Design review of the part built by this model. Coordinates are the model's own, in mm. A direction names the side the tool comes from. Give positions to 0.01 mm unless a question says otherwise; leave off trailing zeros. Order: outer loops, then holes, each group sorted by start corner. A loop starts at its lowest first (then second) coordinate and runs counter-clockwise, first axis right, second up. Notation, with made-up numbers: (33.25, 81.5) -> (40.25, 81.5) arc R15 ccw to (40.25, 105.5) -> close; hole circle Ø8 at (73.5, -18). An arc over 180 degrees is marked (long way). Return JSON: item names as keys, results as strings.
```python
from build123d import *

# Parameters (mm, degrees)
ESTRUSIONE_ESTRUSIONE1_DEPTH      = 30
ESTRUSIONE_ESTRUSIONE1_DEPTH_BACK = 55
SCHIZZO1_R                        = 25
SCHIZZO1_R_2                      = 20
ESTRUSIONE_ESTRUSIONE2_DEPTH      = 10
ESTRUSIONE_ESTRUSIONE3_DEPTH      = 10
ESTRUSIONE_ESTRUSIONE5_DEPTH      = 42.5
TAGLIO_ESTRUSIONE1_DEPTH          = 26.5
SCHIZZO3D5_R                      = 2.5
TAGLIO_ESTRUSIONE2_DEPTH          = 35.5
SCHIZZO3D6_R                      = 4
TAGLIO_ESTRUSIONE3_DEPTH          = 3
ESTRUSIONE_ESTRUSIONE10_DEPTH     = 5
TAGLIO_ESTRUSIONE4_START          = -14
TAGLIO_ESTRUSIONE4_DEPTH          = 14
TAGLIO_ESTRUSIONE7_DEPTH          = 3
ESTRUSIONE_ESTRUSIONE11_START     = 30
ESTRUSIONE_ESTRUSIONE11_OUTLINE_R = 4
ESTRUSIONE_ESTRUSIONE11_DEPTH     = 10
ESTRUSIONE_ESTRUSIONE12_DEPTH     = 10
ESTRUSIONE_ESTRUSIONE13_DEPTH     = 10
ESTRUSIONE_ESTRUSIONE14_DEPTH     = 10
TAGLIO_ESTRUSIONE11_DEPTH         = 80
SCHIZZO3D17_R                     = 4
TAGLIO_ESTRUSIONE12_DEPTH         = 3
TAGLIO_ESTRUSIONE13_START         = 30
TAGLIO_ESTRUSIONE13_OUTLINE_R     = 2.5
TAGLIO_ESTRUSIONE13_DEPTH         = 7
TAGLIO_ESTRUSIONE14_START         = -55
TAGLIO_ESTRUSIONE14_OUTLINE_R     = 25
TAGLIO_ESTRUSIONE14_OUTLINE_R_2   = 20
TAGLIO_ESTRUSIONE14_DEPTH         = 20


# Read off the part's stored shape, not the designer's step: Estrusione-Estrusione11, Taglio-Estrusione13, Taglio-Estrusione14
with BuildPart() as part:
    # Schizzo1 → Estrusione-Estrusione1 (new, two sides: drawn at the far end of the back side and taken through both)
    with BuildSketch(Plane.XY.offset(-ESTRUSIONE_ESTRUSIONE1_DEPTH_BACK)):
        Circle(SCHIZZO1_R)
        Circle(SCHIZZO1_R_2, mode=Mode.SUBTRACT)
    extrude(amount=ESTRUSIONE_ESTRUSIONE1_DEPTH + ESTRUSIONE_ESTRUSIONE1_DEPTH_BACK)

    # Schizzo3D1 → Estrusione-Estrusione2 (add)
    with BuildSketch(Plane(origin=(-37.75, 73.5, 30), x_dir=(0.4568693936855125, -0.889533786381064, 0), z_dir=(0, 0, -1))):
        Polygon((0, 0), (34.493639223, -67.159800872), (75.600538561, -73.870637396), (146.763241471, -37.321085901), (165.255105821, 0), (130.761466598, 67.159800872), (89.654567261, 73.870637396), (18.49186435, 37.321085901), align=None)
    extrude(amount=-ESTRUSIONE_ESTRUSIONE2_DEPTH)

    # Schizzo3D2 → Estrusione-Estrusione3 (add)
    with BuildSketch(Plane(origin=(62.5, 0, 30), x_dir=(-0.9968152785361251, -0.07974522228289001, 0), z_dir=(0, 0, 1))):
        Polygon((0, 0), (0.797452223, 9.968152785), (5.781528616, 9.569426674), (4.984076393, -0.398726111), align=None)
        Polygon((125.39936204, 0), (120.415285647, 0.398726111), (119.617833424, -9.569426674), (124.601909817, -9.968152785), align=None)
    extrude(amount=-ESTRUSIONE_ESTRUSIONE3_DEPTH)

    # Schizzo3D3 → Estrusione-Estrusione5 (add)
    with BuildSketch(Plane(origin=(35.227450684, -68.5, 30), x_dir=(-0.9974912873801348, -0.0707893466612134, 0), z_dir=(0, 0, 1))):
        Polygon((0, 0), (70.278150268, -4.987456437), (70.632097001, 0), (0.353946733, 4.987456437), align=None)
    extrude(amount=-ESTRUSIONE_ESTRUSIONE5_DEPTH)

    # Schizzo3D4 → Taglio-Estrusione1 (cut)
    with BuildSketch(Plane(origin=(32.75, -68.5, -12.5), x_dir=(-1, 0, 0), z_dir=(0, 1, 0))):
        with BuildLine():
            Line((0, 0), (65.5, 0))
            ThreePointArc((65.5, 0), (32.75, 32.75), (0, 0))
        make_face()
    extrude(amount=-TAGLIO_ESTRUSIONE1_DEPTH, mode=Mode.SUBTRACT)

    # Schizzo3D5 → Taglio-Estrusione2 (cut)
    with BuildSketch(Plane(origin=(-52.5, 33.353317087, 40), x_dir=(0.8440673996564301, -0.5362370975951146, 0), z_dir=(0, 0, -1))):
        with Locations(Location((0, 0, 0), (0, 0, 147.572152721))):
            Circle(SCHIZZO3D5_R)
        with Locations(Location((88.627076964, -56.304895247, 0), (0, 0, 147.572152721))):
            Circle(SCHIZZO3D5_R)
        with Locations(Location((124.397648864, 0, 0), (0, 0, 147.572152721))):
            Circle(SCHIZZO3D5_R)
        with Locations(Location((35.7705719, 56.304895247, 0), (0, 0, 147.572152721))):
            Circle(SCHIZZO3D5_R)
    extrude(amount=TAGLIO_ESTRUSIONE2_DEPTH, mode=Mode.SUBTRACT)

    # Schizzo3D6 → Taglio-Estrusione3 (cut)
    with BuildSketch(Plane(origin=(0, 73.5, 40), x_dir=(0, -1, 0), z_dir=(0, 0, -1))):
        with Locations(Location((40.146682913, 52.5, 0), (0, 0, 270))):
            Circle(SCHIZZO3D6_R)
        with Locations(Location((40.146682913, -52.5, 0), (0, 0, 270))):
            Circle(SCHIZZO3D6_R)
        with Locations(Location((106.853317087, -52.5, 0), (0, 0, 270))):
            Circle(SCHIZZO3D6_R)
        with Locations(Location((106.853317087, 52.5, 0), (0, 0, 270))):
            Circle(SCHIZZO3D6_R)
    extrude(amount=TAGLIO_ESTRUSIONE3_DEPTH, mode=Mode.SUBTRACT)

    # Schizzo3D7 → Estrusione-Estrusione10 (add)
    with BuildSketch(Plane(origin=(35.227450684, -73.5, -12.5), x_dir=(-0.8117651174974726, 0, 0.5839840700004706), z_dir=(0, 1, 0))):
        with BuildLine():
            Line((0, 0), (2.011108045, -1.446791734))
            ThreePointArc((2.011108045, -1.446791734), (47.721893936, 6.013037572), (55.181723242, -39.697748319))
            Line((55.181723242, -39.697748319), (57.192831287, -41.144540052))
            Line((57.192831287, -41.144540052), (82.012154262, -6.644522559))
            Line((82.012154262, -6.644522559), (84.059871804, -8.117651175))
            Line((84.059871804, -8.117651175), (89.899712504, 0))
            Line((89.899712504, 0), (28.611446133, 44.090797285))
            Line((28.611446133, 44.090797285), (22.771605433, 35.97314611))
            Line((22.771605433, 35.97314611), (24.819322975, 34.500017494))
            Line((24.819322975, 34.500017494), (0, 0))
        make_face()
    extrude(amount=-ESTRUSIONE_ESTRUSIONE10_DEPTH)

    # Schizzo3D8 → Taglio-Estrusione4 (cut)
    with BuildSketch(Plane(origin=(0, -78.5, 20.25), x_dir=(-0.707106781186551, 0, -0.7071067811865441), z_dir=(0, -1, 0)).offset(TAGLIO_ESTRUSIONE4_START)):
        with BuildLine():
            ThreePointArc((0, 46.315494168), (-0.707106781, -0.707106781), (46.315494168, 0))
            ThreePointArc((46.315494168, 0), (0, 0), (0, 46.315494168))
        make_face()
    extrude(amount=TAGLIO_ESTRUSIONE4_DEPTH, mode=Mode.SUBTRACT)

    # Schizzo3D9 → Taglio-Estrusione7 (cut)
    with BuildSketch(Plane(origin=(35.227450684, -68.5, -12.5), x_dir=(-0.8562730712113632, 0, 0.5165234046180869), z_dir=(0, -1, 0))):
        with BuildLine():
            Line((0, 0), (2.121374306, 1.279661262))
            ThreePointArc((2.121374306, 1.279661262), (13.749394894, 45.407843828), (58.20726047, 35.111944264))
            Line((58.20726047, 35.111944264), (60.328634776, 36.391605526))
            Line((60.328634776, 36.391605526), (82.280879472, 0))
            Line((82.280879472, 0), (21.952244696, -36.391605526))
            Line((21.952244696, -36.391605526), (0, 0))
        make_face()
    extrude(amount=TAGLIO_ESTRUSIONE7_DEPTH, mode=Mode.SUBTRACT)

    # Estrusione-Estrusione11 outline → Estrusione-Estrusione11 (add)
    with BuildSketch(Plane.XY.offset(ESTRUSIONE_ESTRUSIONE11_START)):
        with Locations((52.5, -33.353317087)):
            Circle(ESTRUSIONE_ESTRUSIONE11_OUTLINE_R)
        with Locations((-52.5, -33.353317087)):
            Circle(ESTRUSIONE_ESTRUSIONE11_OUTLINE_R)
    extrude(amount=ESTRUSIONE_ESTRUSIONE11_DEPTH)

    # Schizzo3D11 → Estrusione-Estrusione12 (add)
    with BuildSketch(Plane(origin=(-62.5, -40, 40), x_dir=(0.9979582700578467, -0.06386932928370219, 0), z_dir=(0, 0, -1))):
        Polygon((0, 0), (0.510954634, 7.98366616), (27.158436361, 36.840627497), (26.839089715, 31.850836147), align=None)
        Polygon((102.504285751, 32.018493137), (102.184939104, 27.028701786), (124.744783757, -7.98366616), (125.255738392, 0), align=None)
    extrude(amount=ESTRUSIONE_ESTRUSIONE12_DEPTH)

    # Schizzo3D12 → Estrusione-Estrusione13 (add)
    with BuildSketch(Plane(origin=(-37.75, -78.5, 40), x_dir=(0.9932296706390209, 0.11616721294023631, 0), z_dir=(0, 0, 1))):
        Polygon((0, 0), (-9.932296706, 1.161672129), (-8.770624577, 11.093968836), (1.161672129, 9.932296706), align=None)
        Polygon((74.988840133, -8.770624577), (84.92113684, -9.932296706), (86.082808969, 0), (76.150512263, 1.161672129), align=None)
    extrude(amount=-ESTRUSIONE_ESTRUSIONE13_DEPTH)

    # Schizzo3D15 → Estrusione-Estrusione14 (add)
    with BuildSketch(Plane(origin=(-49.75, -63.712121212, 40), x_dir=(0.9860632358712049, -0.16637095558783233, 0), z_dir=(0, 0, 1))):
        Polygon((0, 0), (4.627662115, -4.074759177), (2.768690441, -4.388409339), (4.432399997, -14.249041698), (98.601439022, 1.639384561), (96.937729467, 11.500016919), (95.078757792, 11.186366757), (98.113291969, 16.553910081), (100.573565494, 1.972126472), (100.906307405, 0), (2.793015436, -16.553910081), (2.460273525, -14.581783609), align=None)
    extrude(amount=-ESTRUSIONE_ESTRUSIONE14_DEPTH)

    # Schizzo3D16 → Taglio-Estrusione11 (cut)
    with BuildSketch(Plane(origin=(-49.75, -80.5, 40), x_dir=(0.9860632358712049, 0.16637095558783233, 0), z_dir=(0, 0, 1))):
        Polygon((0, 0), (1.972126472, -0.332741911), (4.35509632, 13.790870902), (2.793015436, 16.553910081), align=None)
        Polygon((98.113291969, -16.553910081), (96.141165497, -16.22116817), (98.524135346, -2.097555357), (100.906307405, 0), align=None)
    extrude(amount=-TAGLIO_ESTRUSIONE11_DEPTH, mode=Mode.SUBTRACT)

    # Schizzo3D17 → Taglio-Estrusione12 (cut)
    with BuildSketch(Plane(origin=(0, -80.5, 40), x_dir=(-0.9847878761773714, 0.17376086709631217, 0), z_dir=(0, 0, -1))):
        with Locations(Location((41.215356952, 0, 0), (0, 0, 169.993443701))):
            Circle(SCHIZZO3D17_R)
        with Locations(Location((-38.726539684, 14.10534554, 0), (0, 0, 169.993443701))):
            Circle(SCHIZZO3D17_R)
    extrude(amount=TAGLIO_ESTRUSIONE12_DEPTH, mode=Mode.SUBTRACT)

    # Taglio-Estrusione13 outline → Taglio-Estrusione13 (cut)
    with BuildSketch(Plane.XY.offset(TAGLIO_ESTRUSIONE13_START)):
        with Locations((-40.588383838, -73.338383838)):
            Circle(TAGLIO_ESTRUSIONE13_OUTLINE_R)
        with Locations((40.588383838, -73.338383838)):
            Circle(TAGLIO_ESTRUSIONE13_OUTLINE_R)
    extrude(amount=TAGLIO_ESTRUSIONE13_DEPTH, mode=Mode.SUBTRACT)

    # Taglio-Estrusione14 outline → Taglio-Estrusione14 (cut)
    with BuildSketch(Plane.XY.offset(TAGLIO_ESTRUSIONE14_START)):
        Circle(TAGLIO_ESTRUSIONE14_OUTLINE_R)
        Circle(TAGLIO_ESTRUSIONE14_OUTLINE_R_2, mode=Mode.SUBTRACT)
    extrude(amount=TAGLIO_ESTRUSIONE14_DEPTH, mode=Mode.SUBTRACT)


solid = part.part
```
Item 1: Mouldability with a two-part tool opening along Y and no side actions: class faces 1 (the face through (52, 36, 37)), 2 (the face through (47.75, -73, 35)), 3 (the face through (1, -80.5, 35)) as released by +Y, released by -Y, zero draft, split by the parting line, or undercut.
Result set:
{"face 1": "undercut", "face 2": "zero draft", "face 3": "released by -Y"}
Item 2: Add section A-A (z = 26). Give the boundary of the cut face in (x, y).
Result set:
{"outline": "(-62.5, -10) -> (-57.5, -10) -> (-57.5, 0) -> (-62.5, 0) -> close; (-35.23, -78.5) -> (35.23, -78.5) -> (35.23, -71.5) -> (-35.23, -71.5) -> close; circle Ø50 at (0, 0); (57.5, -10) -> (62.5, -10) -> (62.5, 0) -> (57.5, 0) -> close; hole circle Ø40 at (0, 0)"}
Item 3: Wall thickness on L1, parallel to Y at x = 0, z = -3; L2, parallel to Z at x = 25, y = 2; L3, parallel to Y at x = 34, z = 29: over which ranges is each line inside the solid? List them lowest first. Write a range as [from, to].
Result set:
{"L1": "y = [-25, -20], [20, 25]", "L2": "z = [30, 40]", "L3": "y = [-78.5, -71.5]"}
Item 4: Add section C-C (z = 2). Give the boundary of the cut face in (x, y), plus the area to 3 significant figures.
Result set:
{"outline": "(-35.23, -78.5) -> (-29.85, -78.5) -> (-29.85, -71.5) -> (-35.23, -71.5) -> close; circle Ø50 at (0, 0); (29.85, -78.5) -> (35.23, -78.5) -> (35.23, -71.5) -> (29.85, -71.5) -> close; hole circle Ø40 at (0, 0)", "area": "782 mm^2"}
Item 5: Add section D-D (x = 15). Give the boundary of the cut face in (y, z).
Result set:
{"outline": "(-80.5, 30) -> (-78.5, 30) -> (-78.5, 17.61) -> (-71.5, 17.61) -> (-71.5, 30) -> (-20, 30) -> (-20, -35) -> (-13.23, -35) -> (-13.23, 30) -> (13.23, 30) -> (13.23, -35) -> (20, -35) -> (20, 30) -> (73.5, 30) -> (73.5, 40) -> (-80.5, 40) -> close"}
Item 6: Machinability: for faces 4 (the face through (-53, 36, 37)), 5 (the face through (-4.336, -19.524, -2.955)), 6 (the face through (60, -5, 20)), 7 (the face through (-1, -78.5, 23)), 8 (the face through (60, -10, 25)), which of the approach directions +Z, -Z, +X, -X, +Y, -Y give a long, thin tool a straight path to every point of the face, cutting with its end or side? Answer none if there is none.
Result set:
{"face 4": "+Z", "face 5": "-Z", "face 6": "-Z, +X, +Y, -Y", "face 7": "-Z, +X, -X, -Y", "face 8": "-Z, +X, -Y"}
Item 7: Add section B-B (x = 52.5). Give the boundary of the cut face in (y, z), plus the area to 3 significant figures.
Result set:
{"outline": "(-60.32, 30) -> (30.85, 30) -> (30.85, 37) -> (29.35, 37) -> (29.35, 40) -> (-60.32, 40) -> close; (35.85, 30) -> (53.54, 30) -> (53.54, 40) -> (37.35, 40) -> (37.35, 37) -> (35.85, 37) -> close", "area": "1,080 mm^2"}
Item 8: For pin 1 (1.6 mm diameter, centred on y = -72.5, z = 0.5, fed in from -X); pin 2 (1.5 mm diameter, centred on x = 61, z = 24, fed in from +Y); pin 3 (3 mm diameter, centred on x = 52.5, y = 33.35, fed in from -Z); pin 4 (4 mm diameter, centred on x = 60.5, z = 23.5, fed in from -Y), all flat-tipped, find the tip position at first contact; note any pin that passes through.
Result set:
{"pin 1": "stops at x = -35.23", "pin 2": "stops at y = 0", "pin 3": "passes through", "pin 4": "stops at y = -10"}
